Source: three-view drawing plus pictorial views. Frame: mm from the lowest corner of the part. A direction names the side the tool comes from. Coordinates: 2 decimals unless noted, no trailing zeros. Write each loop counter-clockwise with the first axis right and the second up, starting at its lowest first coordinate (ties: lowest second). Pieces come first, ordered by that corner, then holes. Notation, with made-up numbers: (-2.5, 35) - (23.5, 35) arc R12 cw to (23.5, 47) - close; hole circle Ø1 at (63.5, -26.75). An arc over 180 degrees is marked (long way). One line per item, written item: value.
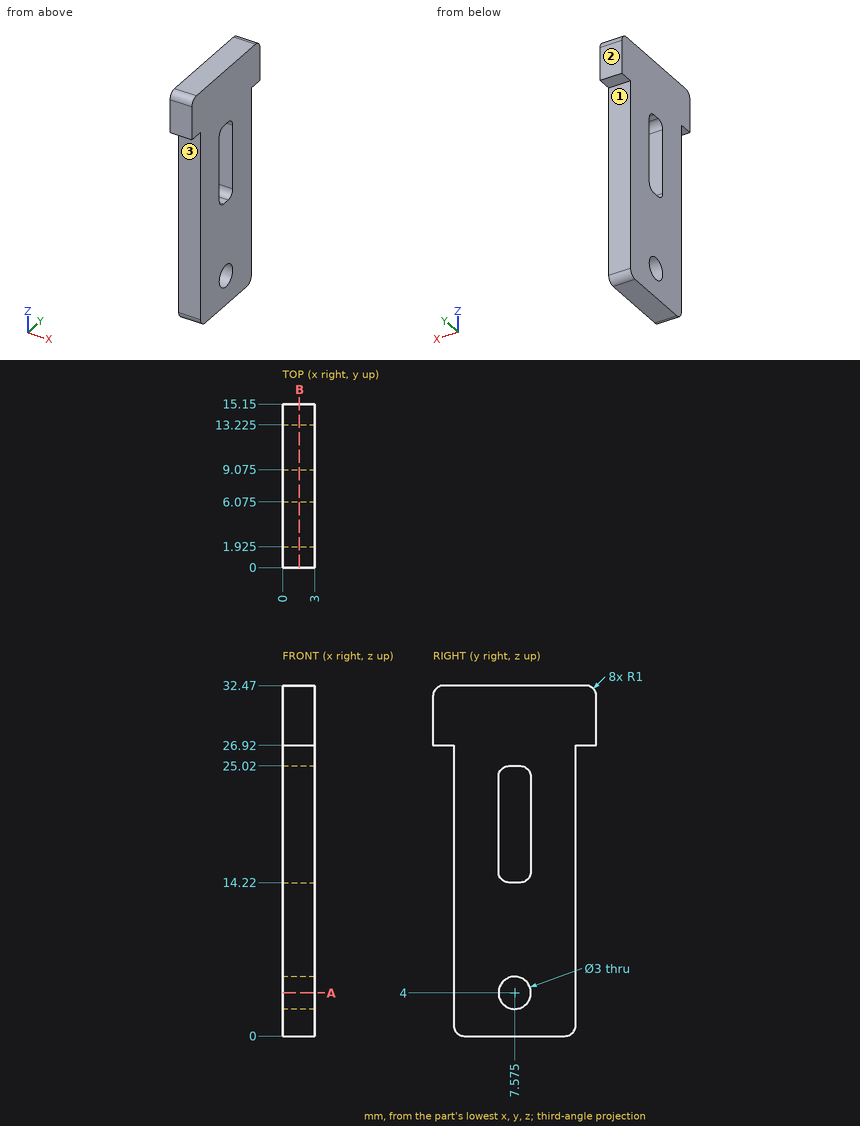
1) Material intervals for line 1 (Z direction, x = 2.2, y = 7.5); line 2 (Z direction, x = 2.5, y = 6.5); line 3 (Y direction, x = 0.85, z = 12.5) (3 decimals), sorted ascending.
Values found:
line 1: 0 to 2.5, 5.5 to 14.22, 25.02 to 32.47
line 2: 0 to 2.95, 5.05 to 14.4, 24.84 to 32.47
line 3: 1.925 to 13.225
2) Reachability of the marked faces 1, 2 and 3 from +Z, -Z, +X, -X, +Y, -Y: full face, straight path, thin tool, end or side. Return the list, or none.
Values found:
face 1: -Z, +X, -X, +Y
face 2: +Z, -Z, +X, -X, +Y
face 3: -Z, +X, -X, -Y
3) Section query A-A on z = 4. Output: boundary loops of the cut face in (x, y) (3 decimals).
Values found:
outline: (0, 1.925) - (3, 1.925) - (3, 6.075) - (0, 6.075) - close; (0, 9.075) - (3, 9.075) - (3, 13.225) - (0, 13.225) - close
4) Section query B-B on x = 1.55. Output: boundary loops of the cut face in (y, z) (3 decimals), then the cut area to 3 significant figures.
Values found:
outline: (0, 26.92) - (1.925, 26.92) - (1.925, 1) arc R1 ccw to (2.925, 0) - (12.225, 0) arc R1 ccw to (13.225, 1) - (13.225, 26.92) - (15.15, 26.92) - (15.15, 31.47) arc R1 ccw to (14.15, 32.47) - (1, 32.47) arc R1 ccw to (0, 31.47) - close; hole circle Ø3 at (7.575, 4); hole (6.075, 15.22) arc R1 ccw to (7.075, 14.22) - (8.075, 14.22) arc R1 ccw to (9.075, 15.22) - (9.075, 24.02) arc R1 ccw to (8.075, 25.02) - (7.075, 25.02) arc R1 ccw to (6.075, 24.02) - close
area: 349 mm2
5) Contact query for flat-ended pins moving along their axis: P1, Ø0.6, axis at x = 2, y = 0.5, coming from the -Z side; P2, Ø1.5, axis at x = 1, z = 15.5, coming from the -Y side (3 decimals). Output: stop coordinate, or through.
Values found:
P1: z = 26.92
P2: y = 1.925
